Work out the finished part from the listing and answer in its coordinate system (mm). Face numbers are marked on the shaded views. Give positions to 0.01 mm unless a question says otherwise; leave off trailing zeros. Loops run counter-clockwise (first coordinate to the right, second up) from the corner with the lowest first, then second, coordinate; pieces in that order, holes last. Notation, with made-up numbers: M 24,30 L 42,30 A15 cw 42,39 Z; hole C 55.5,35 d3. An arc over 180 degrees is marked long. Write item = value, one per line. Start each with the question number.
1. Section A-A on x = 150 is taken. Determine the outline of the cut face in (y, z).
2. The mould has two halves that part along Y. Classify the marked faces 1 and 2: released by +Y, released by -Y, zero draft, split by the parting line, or undercut.
3. Section B-B on x = 105 is taken. Determine the outline of the cut face in (y, z).
4. Consider L1, parallel to X at y = -26, z = 2.85; L2, parallel to X at y = 5, z = 2.5; L3, parallel to X at y = -29.35, z = 8. Determine where each line is inside the solid, lowest interval first. Write a range as [from, to].
5. Flat-ended cylindrical pins translate along their axes: pin 1 Ø2.5 at (x, z) = (90, 8) entering from +Y; pin 2 Ø1.2 at (y, z) = (29.5, 6.5) entering from +X; pin 3 Ø10 at (x, y) = (-29, -22) entering from +Z. Find the tip coordinate at first contact, or state that the pin passes through.
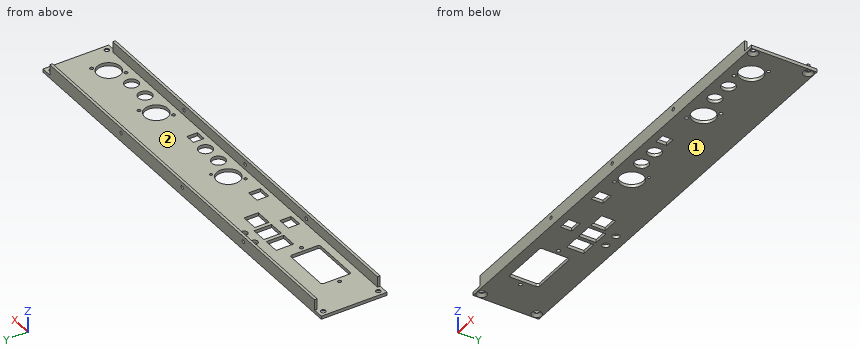
```python
from build123d import *

# Parameters (mm, degrees)
SKETCH_1_W                  = 410
SKETCH_1_H                  = 62
EXTRUDE_1_DEPTH             = 3
HOLE_WIZARD_M4_1_AT_2_COUNT = 2
HOLE_WIZARD_M4_1_AT_2_PITCH = 52
HOLE_WIZARD_M4_1_AT_3_COUNT = 2
HOLE_WIZARD_M4_1_AT_3_PITCH = 403.365838911
HOLE_WIZARD_M4_1_AT_4_COUNT = 2
HOLE_WIZARD_M4_1_AT_4_PITCH = 400
SKETCH_5_W                  = 390
SKETCH_5_H                  = 2.5
EXTRUDE_2_DEPTH             = 10
SKETCH_6_R                  = 1.7
SKETCH_6_W                  = 15.9
SKETCH_6_H                  = 13.5
SKETCH_6_W_2                = 14.5
SKETCH_6_H_2                = 16.5
SKETCH_6_W_3                = 12.3
SKETCH_6_H_3                = 10.7
SKETCH_6_H_4                = 11.1
SKETCH_6_R_2                = 11
SKETCH_6_R_3                = 1.217933171
SKETCH_6_R_4                = 6.4
SKETCH_6_R_5                = 1.507896367
SKETCH_6_W_4                = 9.75
SKETCH_6_H_5                = 10.05
SKETCH_6_R_6                = 1.6
SKETCH_6_R_7                = 3.25
CUT_EXTRUDE_1_DEPTH         = 10
HOLE_WIZARD_M4_1_2_D        = 3.3


with BuildPart() as part:
    # 草圖1 → 填料-伸長1 (new body)
    with BuildSketch(Plane.XY):
        Rectangle(SKETCH_1_W, SKETCH_1_H)
    extrude(amount=EXTRUDE_1_DEPTH)

    # 草圖2 → Hole Wizard M4 _1 (revolve, cut)
    with BuildSketch(Plane(origin=(-200, 26, 0), x_dir=(0, 1, 0), z_dir=(1, 0, 0))):
        Polygon((0, 0), (0, 3), (2.25, 3), (2.25, 2.45), (4.7, 0), align=None)
    hole_wizard_m4_1 = revolve(axis=Axis((-200, 26, -6.35), (0, 0, 1)), mode=Mode.SUBTRACT)

    # Hole Wizard M4 _1 at 2: Hole Wizard M4 _1 ×2
    with Locations(*[(0, -i * HOLE_WIZARD_M4_1_AT_2_PITCH, 0) for i in range(1, HOLE_WIZARD_M4_1_AT_2_COUNT)]):
        add(hole_wizard_m4_1, mode=Mode.SUBTRACT)

    # Hole Wizard M4 _1 at 3: Hole Wizard M4 _1 ×2
    with Locations(*[Vector(0.991655617, -0.12891523, 0) * (i * HOLE_WIZARD_M4_1_AT_3_PITCH) for i in range(1, HOLE_WIZARD_M4_1_AT_3_COUNT)]):
        add(hole_wizard_m4_1, mode=Mode.SUBTRACT)

    # Hole Wizard M4 _1 at 4: Hole Wizard M4 _1 ×2
    with Locations(*[(i * HOLE_WIZARD_M4_1_AT_4_PITCH, 0, 0) for i in range(1, HOLE_WIZARD_M4_1_AT_4_COUNT)]):
        add(hole_wizard_m4_1, mode=Mode.SUBTRACT)

    # 草圖5 → 填料-伸長2 (add)
    with BuildSketch(Plane.XY.offset(3)):
        with Locations((0, 29.75)):
            Rectangle(SKETCH_5_W, SKETCH_5_H)
        with Locations((0, -29.75)):
            Rectangle(SKETCH_5_W, SKETCH_5_H)
    extrude(amount=EXTRUDE_2_DEPTH)

    # 草圖6 → 除料-伸長1 (cut)
    with BuildSketch(Plane.XY.offset(3)):
        with BuildLine():
            ThreePointArc((-167.568, 4.65), (-166.982213562, 6.064213562), (-165.568, 6.65))
            Line((-165.568, 6.65), (-122.468, 6.65))
            ThreePointArc((-122.468, 6.65), (-121.053786438, 6.064213562), (-120.468, 4.65))
            Line((-120.468, 4.65), (-120.468, -19.45))
            ThreePointArc((-120.468, -19.45), (-121.053786438, -20.864213562), (-122.468, -21.45))
            Line((-122.468, -21.45), (-165.568, -21.45))
            ThreePointArc((-165.568, -21.45), (-166.982213562, -20.864213562), (-167.568, -19.45))
            Line((-167.568, -19.45), (-167.568, 4.65))
        make_face()
        with Locations((-172.018, -7.4)):
            Circle(SKETCH_6_R)
        with Locations((-116.018, -7.4)):
            Circle(SKETCH_6_R)
        with Locations((-64.268, 1.95)):
            Rectangle(SKETCH_6_W, SKETCH_6_H)
        with Locations((-83.018, 3.45)):
            Rectangle(SKETCH_6_W_2, SKETCH_6_H_2)
        with Locations((-101.018, 3.45)):
            Rectangle(SKETCH_6_W_2, SKETCH_6_H_2)
        with Locations((-81.018, -18.65)):
            Rectangle(SKETCH_6_W_3, SKETCH_6_H_3)
        with Locations((-34.9934, -18.85)):
            Rectangle(SKETCH_6_W_3, SKETCH_6_H_4)
        with Locations((-1.0082, -11.9)):
            Circle(SKETCH_6_R_2)
        with Locations((8.8918, -2)):
            Circle(SKETCH_6_R_3)
        with Locations((22.0042, -17.35)):
            Circle(SKETCH_6_R_4)
        with Locations((-10.9082, -21.8)):
            Circle(SKETCH_6_R_5)
        with Locations((59.012, -19.375)):
            Rectangle(SKETCH_6_W_4, SKETCH_6_H_5)
        with Locations((41.0034, -17.35)):
            Circle(SKETCH_6_R_4)
        with Locations((105, -11.9)):
            Circle(SKETCH_6_R_2)
        with Locations((130, -17.35)):
            Circle(SKETCH_6_R_4)
        with Locations((150, -17.35)):
            Circle(SKETCH_6_R_4)
        with Locations((175, -11.9)):
            Circle(SKETCH_6_R_2)
        with Locations((184.9, -2)):
            Circle(SKETCH_6_R_6)
        with Locations((165.1, -21.8)):
            Circle(SKETCH_6_R_6)
        with Locations((114.9, -2)):
            Circle(SKETCH_6_R_6)
        with Locations((95.1, -21.8)):
            Circle(SKETCH_6_R_6)
        with Locations((-74.365709963, 20.2)):
            Circle(SKETCH_6_R_7)
        with Locations((-89.365709963, 20.2)):
            Circle(SKETCH_6_R_7)
    extrude(amount=-CUT_EXTRUDE_1_DEPTH, mode=Mode.SUBTRACT)

    # Hole Wizard M4 _1 2 (through all)
    with Locations(Plane(origin=(0, 31, 0), x_dir=(1, 0, 0), z_dir=(0, 1, 0))):
        with Locations((0, -8), (-90, -8), (90, -8)):
            Hole(HOLE_WIZARD_M4_1_2_D / 2)


solid = part.part
```
Verdict:
q1.outline = M -31,0 L -23.75,0 L -23.75,3 L -28.5,3 L -28.5,13 L -31,13 Z; M -10.95,0 L 31,0 L 31,13 L 28.5,13 L 28.5,3 L -10.95,3 Z
q2.face_1 = zero draft
q2.face_2 = undercut
q3.outline = M -31,0 L -22.9,0 L -22.9,3 L -28.5,3 L -28.5,13 L -31,13 Z; M -0.9,0 L 31,0 L 31,13 L 28.5,13 L 28.5,3 L -0.9,3 Z
q4.L1 = [-205, -202.25], [-197.75, 197.75], [202.25, 205]
q4.L2 = [-205, -167.54], [-120.5, -108.27], [-93.77, -90.27], [-75.77, -72.22], [-56.32, 205]
q4.L3 = [-195, -91.65], [-88.35, -1.65], [1.65, 88.35], [91.65, 195]
q5.pin_1 = through
q5.pin_2 = 195
q5.pin_3 = 3
